Geometry check sheet. Reference: the model listing, model coordinates, mm. A direction names the side the tool comes from. Round coordinates to 2 decimals unless told otherwise and drop trailing zeros. Order: outer loops, then holes, each group sorted by start corner. A loop starts at its lowest first (then second) coordinate and runs counter-clockwise, first axis right, second up.
(1) Sectioned sample at A-A (y = 7.25). Record the boundary of the cut face in (x, z), plus the area to 3 significant figures.
(2) Release check for a two-part mould opening along Y. For faces 1 (the face through (0, 0, -12.7)), 2 (the face through (24, -0.1, -5)), 3 (the face through (0, -8.791, 0)) record: +Y half, -Y half, draft (parallel to the pull), parting line (faces both ways), or undercut.
(3) Go/stop test with a flat-tipped pin: pin 1 (2.5 mm diameter, centred on y = 0, z = -6.35, fed in from -X). Record where the tip stops, or that it passes through.
(4) Set-up check for faces 4 (the face through (24, -0.1, 7.7)), 5 (the face through (-24, -0.1, 7.7)), 6 (the face through (0, -8, -12)): record each of +Z, -Z, +X, -X, +Y, -Y from which the full face is reachable in a straight line by a thin tool's end or side.
(5) Material ranges on line 1 along Z through (x, y) = (23, 0); line 2 along Y through (x, z) = (-21.75, -6.35); line 3 along Y through (x, z) = (21.5, 6.5), recorded low to high.
from build123d import *

# Parameters (mm, degrees)
SKETCH1_W                      = 25.4
SKETCH1_H                      = 17.582007
BOSS_EXTRUDE1_DEPTH            = 28.67025
F_6_32_TAPPED_HOLE1_AT_2_COUNT = 2
F_6_32_TAPPED_HOLE1_AT_2_PITCH = 12.7
FILLET1_R                      = 2.54


with BuildPart() as part:
    # Sketch1 → Boss-Extrude1 (new, symmetric)
    with BuildSketch(Plane(origin=(0, 0, 0), x_dir=(0, 0, -1), z_dir=(1, 0, 0))):
        Rectangle(SKETCH1_W, SKETCH1_H)
    extrude(amount=BOSS_EXTRUDE1_DEPTH, both=True)

    # Sketch3 → #6-32 Tapped Hole1 (revolve, cut)
    with BuildSketch(Plane(origin=(28.67025, 0, 6.35), x_dir=(0, 0, -1), z_dir=(0, 1, 0))):
        Polygon((0, 0), (0, 10.21069403), (1.35255, 9.398), (1.35255, 0), align=None)
    f_6_32_tapped_hole1 = revolve(axis=Axis((35.02025, 0, 6.35), (-1, 0, 0)), mode=Mode.SUBTRACT)

    # #6-32 Tapped Hole1 at 2: #6-32 Tapped Hole1 ×2
    with Locations(*[(0, 0, -i * F_6_32_TAPPED_HOLE1_AT_2_PITCH) for i in range(1, F_6_32_TAPPED_HOLE1_AT_2_COUNT)]):
        add(f_6_32_tapped_hole1, mode=Mode.SUBTRACT)

    # Mirror1: #6-32 Tapped Hole1 across plane
    add(f_6_32_tapped_hole1.mirror(Plane(origin=(0, 0, 0), x_dir=(0, 0, 1), z_dir=(1, 0, 0))), mode=Mode.SUBTRACT)

    # Mirror1 copy 1 sketch → Mirror1 copy 1 (revolve, cut)
    with BuildSketch(Plane(origin=(-28.67025, 0, -6.35), x_dir=(0, 0, -1), z_dir=(0, 1, 0))):
        Polygon((0, 0), (0, -10.21069403), (1.35255, -9.398), (1.35255, 0), align=None)
    revolve(axis=Axis((-35.02025, 0, -6.35), (-1, 0, 0)), mode=Mode.SUBTRACT)

    # Fillet1
    fillet1_edges = [part.edges().sort_by_distance(p)[0] for p in [
        (0, -8.7910035, -12.7),
        (0, -8.7910035, 12.7),
        (0, 8.7910035, 12.7),
        (0, 8.7910035, -12.7),
    ]]
    fillet(fillet1_edges, radius=FILLET1_R)


solid = part.part
Answer below:
1. outline: (-28.67, -12.5) - (28.67, -12.5) - (28.67, 12.5) - (-28.67, 12.5) - close
1. area: 1,430 mm2
2. face 1: draft
2. face 2: undercut
2. face 3: -Y half
3. pin 1: stops at x = -19.21
4. face 4: +X
4. face 5: -X
4. face 6: -Z, +X, -X, -Y
5. line 1: z = -12.7 to -7.7, -5 to 5, 7.7 to 12.7
5. line 2: y = -8.79 to -1.35, 1.35 to 8.79
5. line 3: y = -8.79 to -1.34, 1.34 to 8.79
